from build123d import *

# Parameters (mm, degrees)
SKETCH7_R   = 3.5
SKETCH7_R_2 = 3


with BuildPart() as part:
    # Sweep3: sweep along a path in Sketch6
    with BuildLine(Plane(origin=(0, 0, 0), x_dir=(0, 0, -1), z_dir=(1, 0, 0))) as sweep3_path:
        Line((0, 0), (12, 0))
        ThreePointArc((12, 0), (16.233993353, -0.738907352), (19.967422096, -2.868271955))
        ThreePointArc((19.967422096, -2.868271955), (25.605729149, -6.084085697), (32, -7.2))
        Line((32, -7.2), (48, -7.2))
        ThreePointArc((48, -7.2), (55.778174593, -3.978174593), (59, 3.8))
        Line((59, 3.8), (59, 9.8))
    # Sketch7 → Sweep3 (sweep)
    with BuildSketch(Plane.XY):
        Circle(SKETCH7_R)
        Circle(SKETCH7_R_2, mode=Mode.SUBTRACT)
    sweep(path=sweep3_path.line)


solid = part.part
Design review of the part built by this model. Coordinates are the model's own, in mm. A direction names the side the tool comes from. Round coordinates to 2 decimals unless told otherwise and drop trailing zeros. Loops run counter-clockwise (first coordinate to the right, second up) from the corner with the lowest first, then second, coordinate; pieces in that order, holes last. Notation, with made-up numbers: (60.25, 1.5) -> (100.25, 1.5) arc R13 cw to (100.25, 23.5) -> close; hole circle Ø1 at (-23.5, 34.5). An arc over 180 degrees is marked (long way). Use one line per item in the form item = value. Start each with the question number.
Q1. For pin 1 Ø10 at (y, z) = (1, -41) entering from +X; pin 2 Ø2 at (x, z) = (-2, -38) entering from +Y; pin 3 Ø1 at (x, z) = (-0.5, -33) entering from +Y, all flat-tipped, find the tip position at first contact; note any pin that passes through.
Q2. Wall thickness on line 1 along X through (y, z) = (8, -59); line 2 along Z through (x, y) = (0.25, 1.25): over which ranges is each line inside the solid? List them lowest first. Write a range as [from, to].
Q3. Machinability: for faces 1 (the face through (3, 1, 0)), 2 (the face through (0, 7, -62)), 3 (the face through (3.233, 1.341, -6.084)), which of the approach directions +Z, -Z, +X, -X, +Y, -Y give a long, thin tool a straight path to every point of the face, cutting with its end or side? Answer none if there is none.
Q4. We need section D-D on y = 0.75. State how many separate pieces and enclosed holes the cut face has, then the cut area to 3 significant figures.
Q5. We need section B-B on y = 7.5. Give the boundary of the cut face in (x, z).
Q6. Draft analysis for pull direction Z (two halves, no side actions). For faces 4 (the face through (-0.46, -10.67, -40.11)), 5 (the face through (-0.65, -4.27, -40.11)), 6 (the face through (1.615, 6.842, -55.895)), 7 (the face through (-3, 0, -6)), state which applies: +Z half, -Z half, draft (parallel to the pull), parting line (faces both ways), or undercut.
Q7. We need section A-A on x = 0. Give the boundary of the cut face in (y, z).
Q8. We need section C-C on z = -44. Give the boundary of the cut face in (x, y), then the cut area to 3 significant figures.
Calculated:
q1.pin_1 = 1.42
q1.pin_2 = -3.85
q1.pin_3 = -3.7
q2.line_1 = [-3.5, -3], [3, 3.5]
q2.line_2 = [-62.26, -61.76], [-55.59, -55.06], [-20.16, -19.13]
q3.face_1 = +Z, +X, -X, +Y, -Y
q3.face_2 = +Y
q3.face_3 = +Z
q4.separate_pieces = 2
q4.enclosed_holes = 1
q4.area = 35.4 mm²
q5.outline = circle Ø7 at (0, -59); hole circle Ø6 at (0, -59)
q6.face_4 = undercut
q6.face_5 = undercut
q6.face_6 = parting line
q6.face_7 = draft
q7.outline = (-10.7, -48) arc R14.5 ccw to (3.8, -62.5) -> (9.8, -62.5) -> (9.8, -62) -> (3.8, -62) arc R14 cw to (-10.2, -48) -> (-10.2, -32) arc R21.88 cw to (-5.18, -18.06) arc R9.5 ccw to (-3, -12) -> (-3, 0) -> (-3.5, 0) -> (-3.5, -12) arc R9 cw to (-5.57, -17.74) arc R22.38 ccw to (-10.7, -32) -> close; (-4.2, -48) arc R8 ccw to (3.8, -56) -> (9.8, -56) -> (9.8, -55.5) -> (3.8, -55.5) arc R7.5 cw to (-3.7, -48) -> (-3.7, -32) arc R15.38 cw to (-0.17, -22.2) arc R16 ccw to (3.5, -12) -> (3.5, 0) -> (3, 0) -> (3, -12) arc R15.5 cw to (-0.56, -21.88) arc R15.88 ccw to (-4.2, -32) -> close
q8.outline = circle Ø7 at (0, -7.2); hole circle Ø6 at (0, -7.2)
q8.area = 10.2 mm²
